```python
from build123d import *

# Parameters (mm, degrees)
SKETCH1_W           = 15.875
SKETCH1_H           = 31.75
BOSS_EXTRUDE1_DEPTH = 12.7
SKETCH2_R           = 1.5875
BOSS_EXTRUDE2_DEPTH = 25.4


with BuildPart() as part:
    # Sketch1 → Boss-Extrude1 (new body)
    with BuildSketch(Plane(origin=(0, 0, 0), x_dir=(1, 0, 0), z_dir=(0, 1, 0))):
        with Locations((7.9375, 15.875)):
            Rectangle(SKETCH1_W, SKETCH1_H)
    extrude(amount=BOSS_EXTRUDE1_DEPTH)

    # Sketch2 → Boss-Extrude2 (add)
    with BuildSketch(Plane.XZ):
        with Locations((12.7, -3.175)):
            Circle(SKETCH2_R)
        with Locations((12.7, -28.575)):
            Circle(SKETCH2_R)
    extrude(amount=BOSS_EXTRUDE2_DEPTH)


solid = part.part
```
Verification items for the finished model (mm, model axes). A direction names the side the tool comes from. Give positions to 0.01 mm unless a question says otherwise; leave off trailing zeros. Loops run counter-clockwise (first coordinate to the right, second up) from the corner with the lowest first, then second, coordinate; pieces in that order, holes last.
1. Set-up check for faces 1 (the cylindrical face through (13.553, -12.522, -27.236)), 2 (the flat face through (0, 6, -16)): record each of +Z, -Z, +X, -X, +Y, -Y from which the full face is reachable in a straight line by a thin tool's end or side.
2. Section check A-A, the plane x = 12.7. Enter the section's corners in (y, z), then the cut area to 3 significant figures.
3. Section check B-B, the plane z = -9. Enter the section's corners in (x, y) (3 decimals).
4. Go/stop test with flat-tipped pins: pin 1 Ø5 at (x, z) = (3.5, -3.5) entering from -Y; pin 2 Ø6 at (y, z) = (-20.5, -28) entering from +X. Record where each tip stops, or that it passes through.
5. Section check D-D, the plane x = 7.5. Enter the section's corners in (y, z).
6. Thickness scan on line 1 (Y direction, x = 3.75, z = -1.5); line 2 (Z direction, x = 12.5, y = -13.5); line 3 (X direction, y = -14.5, z = -4). Record the ranges inside material, lowest first.
7. Mould release check, pull along Z, two halves, no side actions. Record for faces 3 (the cylindrical face through (14.166, -12.522, -3.783)), 4 (the flat face through (15.875, 6, -16)), 5 (the flat face through (8, 6, 0)): released by +Z, released by -Z, zero draft, split by the parting line, or undercut.
8. Section check C-C, the plane y = -23. Enter the section's corners in (x, z) (1 decimal), then the cut area to 3 significant figures.
Geometry says:
1. face 1: -Y
1. face 2: +Z, -Z, -X, +Y, -Y
2. outline: (-25.4, -30.16) - (0, -30.16) - (0, -31.75) - (12.7, -31.75) - (12.7, 0) - (0, 0) - (0, -1.59) - (-25.4, -1.59) - (-25.4, -4.76) - (0, -4.76) - (0, -26.99) - (-25.4, -26.99) - close
2. area: 565 mm2
3. outline: (0, 0) - (15.875, 0) - (15.875, 12.7) - (0, 12.7) - close
4. pin 1: stops at y = 0
4. pin 2: stops at x = 14.29
5. outline: (0, -31.75) - (12.7, -31.75) - (12.7, 0) - (0, 0) - close
6. line 1: y = 0 to 12.7
6. line 2: z = -30.15 to -27, -4.75 to -1.6
6. line 3: x = 11.34 to 14.06
7. face 3: undercut
7. face 4: zero draft
7. face 5: released by +Z
8. outline: circle Ø3.2 at (12.7, -28.6); circle Ø3.2 at (12.7, -3.2)
8. area: 15.8 mm2
